```python
from build123d import *

# Parameters (mm, degrees)
SKETCH15_R           = 10
BOSS_EXTRUDE11_DEPTH = 80
SKETCH16_R           = 5.3
CUT_EXTRUDE1_DEPTH   = 70
SKETCH18_R           = 5
BOSS_EXTRUDE14_DEPTH = 70


with BuildPart() as part:
    # Sketch15 → Boss-Extrude11 (new body)
    with BuildSketch(Plane(origin=(0, 0, 0), x_dir=(1, 0, 0), z_dir=(0, 1, 0))):
        Circle(SKETCH15_R)
    extrude(amount=BOSS_EXTRUDE11_DEPTH)

    # Sketch16 → Cut-Extrude1 (cut)
    with BuildSketch(Plane(origin=(0, 80, 0), x_dir=(1, 0, 0), z_dir=(0, 1, 0))):
        Circle(SKETCH16_R)
    extrude(amount=-CUT_EXTRUDE1_DEPTH, mode=Mode.SUBTRACT)

    # Sketch18 → Boss-Extrude14 (add)
    with BuildSketch(Plane.XZ):
        Circle(SKETCH18_R)
    extrude(amount=BOSS_EXTRUDE14_DEPTH)


solid = part.part
```
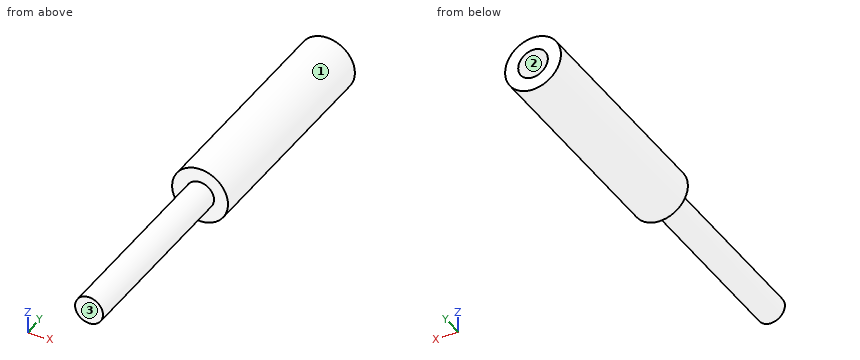
Geometry: final body of the model. Coordinates: model frame, mm. Face numbers are marked on the shaded views. Give positions to 0.01 mm unless a question says otherwise; leave off trailing zeros. Loops run counter-clockwise (first coordinate to the right, second up) from the corner with the lowest first, then second, coordinate; pieces in that order, holes last. Notation, with made-up numbers: (35.5, 65) - (49.5, 65) arc R24 ccw to (49.5, 97) - close; hole circle Ø5 at (-22.5, -5). An arc over 180 degrees is marked (long way). Answer as CSV lines item,"result". Start each with the question number.
(1) Section query D-D (y = 42.5). Output: boundary loops of the cut face in (x, z), and give its area (3 significant figures).
(2) Pin query (flat end, axial travel): P1, Ø3, axis at x = 1.5, z = -2, coming from the +Y side; P2, Ø2, axis at x = 5.5, y = 39.5, coming from the +Z side; P3, Ø1, axis at x = -5.5, y = 11.5, coming from the -Z side. Return the tip coordinate at first contact, or that it passes through.
(3) Section query C-C (y = -4). Output: boundary loops of the cut face in (x, z).
(4) Ray query, line 1 along X through (y, z) = (47, 0); line 2 along Y through (x, z) = (-0.5, -6.5). Return the intervals inside material, ascending. Write a range as [from, to].
(5) Section query B-B (x = -0.5). Output: boundary loops of the cut face in (y, z).
(6) Mould query, pull axis X, two halves, no side actions, for the marked faces 1, 2 and 3. Classes: +X half, -X half, draft (parallel to the pull), parting line (faces both ways), or undercut.
(7) Section query A-A (z = 0). Output: boundary loops of the cut face in (x, y).
Worked answers:
1,outline,"circle Ø20 at (0, 0); hole circle Ø10.6 at (0, 0)"
1,area,"226 mm^2"
2,P1,"stops at y = 10"
2,P2,"stops at z = 8.93"
2,P3,"stops at z = -8.66"
3,outline,"circle Ø10 at (0, 0)"
4,line 1,"x = [-10, -5.3], [5.3, 10]"
4,line 2,"y = [0, 80]"
5,outline,"(-70, -4.97) - (0, -4.97) - (0, -9.99) - (80, -9.99) - (80, -5.28) - (10, -5.28) - (10, 5.28) - (80, 5.28) - (80, 9.99) - (0, 9.99) - (0, 4.97) - (-70, 4.97) - close"
6,face 1,"parting line"
6,face 2,"undercut"
6,face 3,"draft"
7,outline,"(-10, 0) - (-5, 0) - (-5, -70) - (5, -70) - (5, 0) - (10, 0) - (10, 80) - (5.3, 80) - (5.3, 10) - (-5.3, 10) - (-5.3, 80) - (-10, 80) - close"
